Design review of the part built by this model. Coordinates are the model's own, in mm. A direction names the side the tool comes from. Coordinates: 2 decimals unless noted, no trailing zeros. Write each loop counter-clockwise with the first axis right and the second up, starting at its lowest first coordinate (ties: lowest second). Pieces come first, ordered by that corner, then holes. Notation, with made-up numbers: M 52.25,69 L 88.25,69 A12 cw 88.25,78 Z; hole C 9.25,14.5 d7. An arc over 180 degrees is marked long. Write item = value, one per line.
Autodesk Inventor part; units mm, degrees
ref_plane "YZ Plane" through (0, 0, 0) normal (1, 0, 0) x (0, 1, 0)
ref_plane "XZ Plane" through (0, 0, 0) normal (0, 1, 0) x (-1, 0, 0)
ref_plane "XY Plane" through (0, 0, 0) normal (0, 0, 1) x (1, 0, 0)
sketch "Náčrt1" plane through (0, 0, 0) normal (0, 0, 1) x (1, 0, 0)
  line L0 (0, 0) -> (0, 31)
  circle A0 centre (0, 31) radius 1.825
  circle A1 centre (0, 0) radius 1.825
  arc A2 (3.1429, 28.5257) -> (-3.1429, 28.5257) centre (0, 31) ccw
  arc A3 (-3.1429, 2.4743) -> (3.1429, 2.4743) centre (0, 0) ccw
  line L1 (0, 31) -> (-5.5, 31)
  line L2 (-5.5, 31) -> (-5.5, 26.67)
  arc A4 (-2.5003, 26.6349) -> (-3.1429, 28.5257) centre (-5.5, 26.67) ccw
  line L3 (-2.5003, 4.2949) -> (-2.5003, 15.5)
  arc A5 (3.1429, 28.5257) -> (2.5003, 26.6349) centre (5.5, 26.67) ccw
  arc A6 (-3.1429, 2.4743) -> (-2.5003, 4.3651) centre (-5.5, 4.33) ccw
  arc A7 (2.5003, 4.3651) -> (3.1429, 2.4743) centre (5.5, 4.33) ccw
  line L4 (2.5003, 26.6349) -> (2.5003, 4.3651)
  line L5 (-2.5003, 26.6349) -> (-2.5003, 15.5)
  dimension "d0" = 31
  dimension "d1" = 3.65
  dimension "d2" = 3.65
  dimension "d3" = 8
  dimension "d4" = 8
  dimension "d7" = 5.5
  dimension "d8" = 4.33
extrude "Vysunutí1" add sketch "Náčrt1" along normal blind 4
properties part number "spojka" material "ABS Plastic"
Q1. Wall thickness on line 1 (X direction, y = 0, z = 3.05) (3 decimals); line 2 (Y direction, x = -1.5, z = 2.2); line 3 (Y direction, x = 1, z = 3.85): over which ranges is each line inside the solid? List them lowest first.
Check result:
line_1 = -4 to -1.825, 1.825 to 4
line_2 = -3.71 to -1.04, 1.04 to 29.96, 32.04 to 34.71
line_3 = -3.87 to -1.53, 1.53 to 29.47, 32.53 to 34.87
Q2. Consider section B-B, the plane x = -0.5. State the section outline as (y, z) points, and give its area (3 significant figures).
Check result:
outline = M -3.97,0 L -1.76,0 L -1.76,4 L -3.97,4 Z; M 1.76,0 L 29.24,0 L 29.24,4 L 1.76,4 Z; M 32.76,0 L 34.97,0 L 34.97,4 L 32.76,4 Z
area = 128 mm²
Q3. The part is to be moulded in two halves that separate along X. For faces 4 (the flat face through (0, 16, 0)), 5 (the flat face through (-2.5, 16, 2)), 6 (the cylindrical face through (1.74, -0.55, 1.97)), say which applies: +X half, -X half, draft (parallel to the pull), parting line (faces both ways), or undercut.
Check result:
face_4 = draft
face_5 = -X half
face_6 = undercut
Q4. Consider section D-D, the plane y = 13. State the section outline as (x, z) points, and give its area (3 significant figures).
Check result:
outline = M -2.5,0 L 2.5,0 L 2.5,4 L -2.5,4 Z
area = 20.0 mm²
Q5. Consider section A-A, the plane y = 31. State the section outline as (x, z) points (3 decimals), and give its area (3 significant figures).
Check result:
outline = M -4,0 L -1.825,0 L -1.825,4 L -4,4 Z; M 1.825,0 L 4,0 L 4,4 L 1.825,4 Z
area = 17.4 mm²
Q6. For P1, Ø1.2, axis at y = 19.5, z = 2.5, coming from the -X side; P2, Ø1.5, axis at x = 3, z = 1, coming from the +Y side, all flat-tipped, find the tip position at first contact; note any pin that passes through.
Check result:
P1 = -2.5
P2 = 34.31
Q7. Consider section C-C, the plane z = 2.2. State the section outline as (x, y) points (3 decimals), and give its area (3 significant figures).
Check result:
outline = M -3.143,2.474 A4 ccw long 3.143,2.474 A3 cw 2.5,4.365 L 2.5,26.635 A3 cw 3.143,28.526 A4 ccw long -3.143,28.526 A3 cw -2.5,26.635 L -2.5,4.295 A3 cw Z; hole C 0,0 d3.65; hole C 0,31 d3.65
area = 198 mm²
Q8. Machinability: for faces 1 (the cylindrical face through (2.655, 27.622, 1.972)), 2 (the cylindrical face through (0, 35, 2)), 3 (the cylindrical face through (-2.67, 3.34, 1.97)), which of the approach directions +Z, -Z, +X, -X, +Y, -Y give a long, thin tool a straight path to every point of the face, cutting with its end or side? Answer none if there is none.
Check result:
face_1 = +Z, -Z, +X
face_2 = +Z, -Z
face_3 = +Z, -Z, -X
